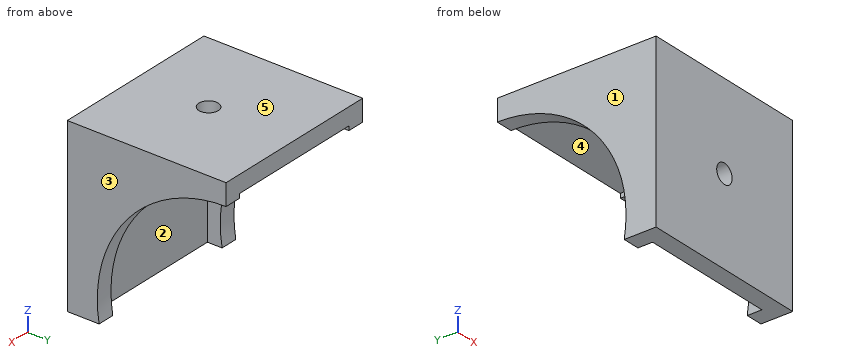
from build123d import *

# Parameters (mm, degrees)
CYLINDER004_R     = 30
CYLINDER004_DEPTH = 40
CYLINDER005_R     = 2.25
CYLINDER005_DEPTH = 20
CYLINDER006_R     = 2.25
CYLINDER006_DEPTH = 20
BOX004_W          = 32
BOX004_H          = 40
BOX004_DEPTH      = 40
BOX003_W          = 40
BOX003_H          = 37
BOX003_DEPTH      = 40


with BuildPart() as cylinder004:
    # Cylinder004 → Cylinder004 (new body)
    with BuildSketch(Plane(origin=(0, 37, 5), x_dir=(0, 0, -1), z_dir=(1, 0, 0))):
        Circle(CYLINDER004_R)
    extrude(amount=CYLINDER004_DEPTH)


with BuildPart() as cylinder005:
    # Cylinder005 → Cylinder005 (new body)
    with BuildSketch(Plane(origin=(20, 10, 20), x_dir=(1, 0, 0), z_dir=(0, -1, 0))):
        Circle(CYLINDER005_R)
    extrude(amount=CYLINDER005_DEPTH)


with BuildPart() as cylinder006:
    # Cylinder006 → Cylinder006 (new body)
    with BuildSketch(Plane(origin=(20, 17, 30), x_dir=(1, 0, 0), z_dir=(0, 0, 1))):
        Circle(CYLINDER006_R)
    extrude(amount=CYLINDER006_DEPTH)


with BuildPart() as fusion002:
    # Box004 → Box004 (new body)
    with BuildSketch(Plane(origin=(4, 4, -4), x_dir=(1, 0, 0), z_dir=(0, 0, 1))):
        with Locations((16, 20)):
            Rectangle(BOX004_W, BOX004_H)
    extrude(amount=BOX004_DEPTH)

    # Fusion002: union Cylinder004, Cylinder005, Cylinder006
    add(cylinder004.part)
    add(cylinder005.part)
    add(cylinder006.part)


with BuildPart() as cut002:
    # Box003 → Box003 (new body)
    with BuildSketch(Plane.XY):
        with Locations((20, 18.5)):
            Rectangle(BOX003_W, BOX003_H)
    extrude(amount=BOX003_DEPTH)

    # Cut002: cut Fusion002
    add(fusion002.part, mode=Mode.SUBTRACT)


with BuildPart() as cut002_1:
    # Cut002 placement: moved
    add(cut002.part.moved(Location((0, 3, 0))))


solid = cut002_1.part
Can you work these out from the model? Positions are in its coordinate system, mm. Face numbers are marked on the shaded views. A direction names the side the tool comes from. Give positions to 0.01 mm unless a question says otherwise; leave off trailing zeros. Loops run counter-clockwise (first coordinate to the right, second up) from the corner with the lowest first, then second, coordinate; pieces in that order, holes last. Notation, with made-up numbers: (85, 60) -> (117, 60) arc R36 ccw to (117, 98) -> close; hole circle Ø11 at (13.25, 22). An arc over 180 degrees is marked (long way). Write item = value, one per line.
1) Thinking about a two-plate mould opening in X: for the marked faces 1, 2 and 3, which applies, released by +X, released by -X, zero draft, split by the parting line, or undercut?
Check result:
face_1 = released by -X
face_2 = undercut
face_3 = released by +X
2) Suppose I cut it at C-C on z = 20. Write out the boundary of the cut face in (x, y), then the cut area to 3 significant figures.
Check result:
outline = (0, 3) -> (17.75, 3) -> (17.75, 7) -> (4, 7) -> (4, 14.02) -> (0, 14.02) -> close; (22.25, 3) -> (40, 3) -> (40, 14.02) -> (36, 14.02) -> (36, 7) -> (22.25, 7) -> close
area = 198 mm2
3) I need wall thicknesses on L1, parallel to Z at x = 20, y = 4.05; L2, parallel to X at y = 7.5, z = 4. Which ranges of each line are inside material? Lowest first, please. Write a range as from..to.
Check result:
L1 = 0..17.75, 22.25..40
L2 = 0..4, 36..40
4) Suppose I cut it at D-D on x = 18.5. Write out the boundary of the cut face in (y, z), then the cut area to 3 significant figures.
Check result:
outline = (3, 0) -> (7, 0) -> (7, 18.32) -> (3, 18.32) -> close; (3, 21.68) -> (7, 21.68) -> (7, 36) -> (18.32, 36) -> (18.32, 40) -> (3, 40) -> close; (21.68, 36) -> (40, 36) -> (40, 40) -> (21.68, 40) -> close
area = 265 mm2
5) Suppose I cut it at A-A on y = 20. Write out the boundary of the cut face in (x, z).
Check result:
outline = (0, 27.36) -> (4, 27.36) -> (4, 36) -> (17.75, 36) -> (17.75, 40) -> (0, 40) -> close; (22.25, 36) -> (36, 36) -> (36, 27.36) -> (40, 27.36) -> (40, 40) -> (22.25, 40) -> close
6) Will these pins go through, and if not, where does the flat tip stop? pin 1 (9.5 mm diameter, centred on x = 14, z = 9.5, fed in from +Y); pin 2 (9.5 mm diameter, centred on x = 14.5, y = 24, fed in from -Z); pin 3 (8 mm diameter, centred on x = 33.5, z = 14.5, fed in from +Y).
Check result:
pin_1 = 7
pin_2 = 36
pin_3 = 12.78
7) For the marked faces 4 and 5, which set-ups out of +Z, -Z, +X, -X, +Y, -Y let a thin tool reach every point of the face, with its end or its side?
Check result:
face_4 = -Z, +Y
face_5 = +Z, +X, -X, +Y, -Y
8) Suppose I cut it at B-B on y = 8. Write out the boundary of the cut face in (x, z).
Check result:
outline = (0, 0) -> (4, 0) -> (4, 36) -> (36, 36) -> (36, 0) -> (40, 0) -> (40, 40) -> (0, 40) -> close
